```python
from build123d import *

# Parameters (mm, degrees)
SKIZZE3_W                       = 5
SKIZZE3_H                       = 23
SCHNITT_LINEAR_AUSTRAGEN1_DEPTH = 9


with BuildPart() as part:
    # Skizze2 → Rotation1 (revolve)
    with BuildSketch(Plane(origin=(0, 0, 0), x_dir=(0, 0, -1), z_dir=(1, 0, 0)), mode=Mode.PRIVATE) as rotation1_sk:
        Polygon((0, 0), (6, 0), (7, 1), (7, 4), (6, 5), (5, 5), (5, 12), (4, 13), (0, 13), align=None)
    revolve(rotation1_sk.sketch.rotate(Axis((0, 0, 0), (0, -1, 0)), 180), axis=Axis((0, 0, 0), (0, -1, 0)))

    # Skizze3 → Schnitt-Linear austragen1 (cut)
    with BuildSketch(Plane(origin=(0, 5, 0), x_dir=(1, 0, 0), z_dir=(0, 1, 0))):
        with Locations((8.5, 0)):
            Rectangle(SKIZZE3_W, SKIZZE3_H)
        with Locations((-8.5, 0)):
            Rectangle(SKIZZE3_W, SKIZZE3_H)
    extrude(amount=-SCHNITT_LINEAR_AUSTRAGEN1_DEPTH, mode=Mode.SUBTRACT)


solid = part.part
```
The model under review builds one solid part; all positions refer to its coordinate system, in mm. A direction names the side the tool comes from. Round coordinates to 2 decimals unless told otherwise and drop trailing zeros. Order: outer loops, then holes, each group sorted by start corner. A loop starts at its lowest first (then second) coordinate and runs counter-clockwise, first axis right, second up.
Item 1: Add section A-A, the plane x = 0. State the section outline as (y, z) points.
Working result:
outline: (0, -6) - (1, -7) - (4, -7) - (5, -6) - (5, -5) - (12, -5) - (13, -4) - (13, 4) - (12, 5) - (5, 5) - (5, 6) - (4, 7) - (1, 7) - (0, 6) - close
Item 2: To check wall thickness, follow probe 1 along Z at (x, y) = (0.25, 1.5); probe 2 along Y at (x, z) = (1.5, 5.25); probe 3 along Y at (x, z) = (-2, -3.5). State the ranges of each line that lie inside material, in increasing order.
Working result:
probe 1: z = -7 to 7
probe 2: y = 0 to 5
probe 3: y = 0 to 12.97
Item 3: Add section C-C, the plane y = 7.5. State the section outline as (x, z) points.
Working result:
outline: circle Ø10 at (0, 0)
Item 4: For pin 1 (1.5 mm diameter, centred on x = 4.5, y = 10.5, fed in from -Z); pin 2 (2 mm diameter, centred on y = 7.5, z = 5, fed in from -X); pin 3 (1 mm diameter, centred on y = 11, z = 1, fed in from +X), all flat-tipped, find the tip position at first contact; note any pin that passes through.
Working result:
pin 1: stops at z = -3.31
pin 2: stops at x = -3
pin 3: stops at x = 4.97
Item 5: Machinability: for faces 1 (the flat face through (6, 3, 0)), 2 (the cylindrical face through (0, 9, -5)), which of the approach directions +Z, -Z, +X, -X, +Y, -Y give a long, thin tool a straight path to every point of the face, cutting with its end or side? Answer none if there is none.
Working result:
face 1: +Z, -Z, +X, +Y, -Y
face 2: +Y
Item 6: Add section B-B, the plane y = 2. State the section outline as (x, z) points, and give its area (3 significant figures).
Working result:
outline: (-6, -3.61) arc R7 ccw to (6, -3.61) - (6, 3.61) arc R7 ccw to (-6, 3.61) - close
area: 144 mm2
Item 7: Add section D-D, the plane y = 4.75. State the section outline as (x, z) points, and give its area (3 significant figures).
Working result:
outline: (-6, -1.75) arc R6.25 ccw to (6, -1.75) - (6, 1.75) arc R6.25 ccw to (-6, 1.75) - close
area: 122 mm2
